For this review, take the finished solid that the model builds, in its own axes (mm). Coordinates: 2 decimals unless noted, no trailing zeros. Write each loop counter-clockwise with the first axis right and the second up, starting at its lowest first coordinate (ties: lowest second). Pieces come first, ordered by that corner, then holes. Notation, with made-up numbers: M 23,-6.5 L 32,-6.5 A23 ccw 32,21.5 Z; hole C 1.5,53.25 d8. An arc over 180 degrees is marked long. Return JSON: item names as keys, results as strings.
```python
from build123d import *

# Parameters (mm, degrees)
F1_DEPTH      = 12.7
F2_R          = 2.3789042868
F3_DEPTH      = 31.75
F3_DEPTH_BACK = 138.176
F4_R          = 5.08
F5_T4_ANGLE   = 90
F5_S5_R       = 2.3789042868
F5_T6_DEPTH   = 6
F5_T10_DEPTH  = 20.32
F5_S11_R      = 2.3789042868
F5_T12_DEPTH  = 12
F5_T16_DEPTH  = 16.390593442
F5_S17_R      = 2.3789042868
F5_T18_DEPTH  = 10
F6_T1_DEPTH   = 113.968887086
F6_T6_ANGLE   = 90.0000000017
F6_S7_R       = 2.3789042868
F6_T8_DEPTH   = 6
F6_T12_DEPTH  = 16.390593442
F6_S13_R      = 2.3789042868
F6_T14_DEPTH  = 10
F7_R          = 1.2458673334
F8_DEPTH      = 25.4
F9_T4_DEPTH   = 16.390593442
F9_S5_R       = 2.3789042868
F9_T6_DEPTH   = 10
F9_T10_DEPTH  = 16.390593442
F9_S11_R      = 2.3789042868
F9_T12_DEPTH  = 10
F9_T16_ANGLE  = 90
F9_S17_R      = 2.3789042868
F9_T18_DEPTH  = 6
F9_T22_DEPTH  = 2.54
F9_S23_R      = 2.3789042868
F9_T24_DEPTH  = 5
F9_T28_ANGLE  = 90.0000000017
F9_S29_R      = 2.3789042868
F9_T30_DEPTH  = 6
F10_R         = 1.24587
F11_DEPTH     = 25.4


# Not quite as in the source:
# - a fillet or chamfer that OpenCascade refuses, or shapes differently, is made with other operations: its cross-section is extruded or revolved along the edge and cut away or added


with BuildPart() as f1:
    # F0 (on Front) → F1 (new body)
    with BuildSketch(Plane.XZ):
        with BuildLine():
            Line((-53.174443543, 7.5021637604), (0, 7.5021637604))
            Line((0, 7.5021637604), (53.174443543, 7.5021637604))
            Line((53.174443543, 7.5021637604), (53.174443543, 16.2727572024))
            Line((53.174443543, 16.2727572024), (27.8020980501, 20.4710588867))
            add(Edge.make_bspline(
                [(27.8020980501, 20.4710588867), (23.5634737704, 22.8817989501), (13.8731335003, 28.3932314282), (12.3127368707, 44.1452356637), (11.4348689094, 53.0072003603)],
                knots=[0, 0, 0, 0, 0.4374071665, 1, 1, 1, 1], degree=3))
            Line((11.4348689094, 53.0072003603), (1.8664607778, 53.0072003603))
            Line((1.8664607778, 53.0072003603), (0, 52.8586618602))
            Line((0, 52.8586618602), (-1.8664607778, 53.0072003603))
            Line((-1.8664607778, 53.0072003603), (-11.4348689094, 53.0072003603))
            add(Edge.make_bspline(
                [(-27.8020980501, 20.4710588867), (-23.5634737704, 22.8817989501), (-13.8731335003, 28.3932314282), (-12.3127368707, 44.1452356637), (-11.4348689094, 53.0072003603)],
                knots=[0, 0, 0, 0, 0.4374071665, 1, 1, 1, 1], degree=3))
            Line((-27.8020980501, 20.4710588867), (-53.174443543, 16.2727572024))
            Line((-53.174443543, 16.2727572024), (-53.174443543, 7.5021637604))
        make_face()
    extrude(amount=F1_DEPTH)

    # F2 (on face) → F3 (join, two sides)
    with BuildSketch(Plane(origin=(-53.174443543, 0, 0), x_dir=(0, -1, 0), z_dir=(-1, 0, 0))) as f3_sk:
        with Locations((6.3686654903, 12.1966870502)):
            Circle(F2_R)
    extrude(amount=F3_DEPTH)
    extrude(f3_sk.sketch, amount=-F3_DEPTH_BACK)

    # F4
    f4_edges = [f1.edges().sort_by_distance(p)[0] for p in [
        (0, 0, 7.502164),
    ]]
    fillet(f4_edges, radius=F4_R)

    # F5: fillet of radius 5.08 on 1 edges, made by hand


with BuildPart() as f5_tool2:
    # F5_s3 → F5_t4 (revolve)
    with BuildSketch(Plane.XZ.offset(5.08)):
        with BuildLine():
            ThreePointArc((-53.174443543, 12.5821637604), (-51.6865459914, 8.9900613119), (-48.094443543, 7.5021637604))
            Line((-48.094443543, 7.5021637604), (-53.174443543, 7.5021637604))
            Line((-53.174443543, 7.5021637604), (-53.174443543, 12.5821637604))
        make_face()
    revolve(axis=Axis((-53.174443543, -5.08, 12.5821637604), (1, 0, 0)), revolution_arc=F5_T4_ANGLE)

    # F5_s5 → F5_t6 (cut, symmetric)
    with BuildSketch(Plane.YZ.offset(-50.6)):
        with Locations((-6.3686654903, 12.1966870502)):
            Circle(F5_S5_R)
    extrude(amount=F5_T6_DEPTH, both=True, mode=Mode.SUBTRACT)


with BuildPart() as f1_1:
    add(f1.part)

    # F5_t1: cut F5_tool2
    add(f5_tool2.part, mode=Mode.SUBTRACT)


with BuildPart() as f5_tool8:
    # F5_s9 → F5_t10 (new body)
    with BuildSketch(Plane.XZ.offset(5.08)):
        with BuildLine():
            ThreePointArc((-48.094443543, 7.5021637604), (-51.6865459914, 8.9900613119), (-53.174443543, 12.5821637604))
            Line((-53.174443543, 12.5821637604), (-53.174443543, 7.5021637604))
            Line((-53.174443543, 7.5021637604), (-48.094443543, 7.5021637604))
        make_face()
    extrude(amount=F5_T10_DEPTH)

    # F5_s11 → F5_t12 (cut, symmetric)
    with BuildSketch(Plane.YZ.offset(-50.6)):
        with Locations((-6.3686654903, 12.1966870502)):
            Circle(F5_S11_R)
    extrude(amount=F5_T12_DEPTH, both=True, mode=Mode.SUBTRACT)


with BuildPart() as f1_2:
    add(f1_1.part)

    # F5_t7: cut F5_tool8
    add(f5_tool8.part, mode=Mode.SUBTRACT)


with BuildPart() as f5_tool14:
    # F5_s15 → F5_t16 (new body)
    with BuildSketch(Plane.XY.offset(28.9727572024)):
        with BuildLine():
            ThreePointArc((-53.174443543, -5.08), (-51.6865459914, -1.4878975516), (-48.094443543, 0))
            Line((-48.094443543, 0), (-53.174443543, 0))
            Line((-53.174443543, 0), (-53.174443543, -5.08))
        make_face()
    extrude(amount=-F5_T16_DEPTH)

    # F5_s17 → F5_t18 (cut, symmetric)
    with BuildSketch(Plane.YZ.offset(-50.6)):
        with Locations((-6.3686654903, 12.1966870502)):
            Circle(F5_S17_R)
    extrude(amount=F5_T18_DEPTH, both=True, mode=Mode.SUBTRACT)


with BuildPart() as f1_3:
    add(f1_2.part)

    # F5_t13: cut F5_tool14
    add(f5_tool14.part, mode=Mode.SUBTRACT)

    # F6: fillet of radius 5.08 on 1 edges, made by hand

    # F6_s2 → F6_t1 (cut)
    with BuildSketch(Plane.YZ.offset(-48.094443543)):
        with BuildLine():
            ThreePointArc((-7.62, 7.5021637604), (-11.2121024484, 8.9900613119), (-12.7, 12.5821637604))
            Line((-12.7, 12.5821637604), (-12.7, 7.5021637604))
            Line((-12.7, 7.5021637604), (-7.62, 7.5021637604))
        make_face()
    extrude(amount=F6_T1_DEPTH, mode=Mode.SUBTRACT)


with BuildPart() as f6_tool4:
    # F6_s5 → F6_t6 (revolve)
    with BuildSketch(Plane.YZ.offset(-48.0944435431)):
        with BuildLine():
            ThreePointArc((-12.7, 12.5821637604), (-11.2121024484, 8.990061312), (-7.62, 7.5021637604))
            Line((-7.62, 7.5021637604), (-12.7, 7.5021637604))
            Line((-12.7, 7.5021637604), (-12.7, 12.5821637604))
        make_face()
    revolve(axis=Axis((-48.0944435431, -12.7, 12.5821637603), (0, 1, 0)), revolution_arc=F6_T6_ANGLE)

    # F6_s7 → F6_t8 (cut, symmetric)
    with BuildSketch(Plane.YZ.offset(-50.6)):
        with Locations((-6.3686654903, 12.1966870502)):
            Circle(F6_S7_R)
    extrude(amount=F6_T8_DEPTH, both=True, mode=Mode.SUBTRACT)


with BuildPart() as f1_4:
    add(f1_3.part)

    # F6_t3: cut F6_tool4
    add(f6_tool4.part, mode=Mode.SUBTRACT)


with BuildPart() as f6_tool10:
    # F6_s11 → F6_t12 (new body)
    with BuildSketch(Plane.XY.offset(28.9727572024)):
        with BuildLine():
            ThreePointArc((-48.094443543, -12.7), (-51.6865459914, -11.2121024484), (-53.174443543, -7.62))
            Line((-53.174443543, -7.62), (-53.174443543, -12.7))
            Line((-53.174443543, -12.7), (-48.094443543, -12.7))
        make_face()
    extrude(amount=-F6_T12_DEPTH)

    # F6_s13 → F6_t14 (cut, symmetric)
    with BuildSketch(Plane.YZ.offset(-50.6)):
        with Locations((-6.3686654903, 12.1966870502)):
            Circle(F6_S13_R)
    extrude(amount=F6_T14_DEPTH, both=True, mode=Mode.SUBTRACT)


with BuildPart() as f1_5:
    add(f1_4.part)

    # F6_t9: cut F6_tool10
    add(f6_tool10.part, mode=Mode.SUBTRACT)

    # F7 (on face) → F8 (cut)
    with BuildSketch(Plane(origin=(-84.924443543, 0, 0), x_dir=(0, -1, 0), z_dir=(-1, 0, 0))):
        with Locations((6.3686654903, 12.1966870502)):
            Circle(F7_R)
    extrude(amount=-F8_DEPTH, mode=Mode.SUBTRACT)

    # F9: fillet of radius 5.08 on 2 edges, made by hand


with BuildPart() as f9_tool2:
    # F9_s3 → F9_t4 (new body)
    with BuildSketch(Plane.XY.offset(12.5821637604)):
        with BuildLine():
            ThreePointArc((53.174443543, -7.62), (51.6865459914, -11.2121024484), (48.094443543, -12.7))
            Line((48.094443543, -12.7), (53.174443543, -12.7))
            Line((53.174443543, -12.7), (53.174443543, -7.62))
        make_face()
    extrude(amount=F9_T4_DEPTH)

    # F9_s5 → F9_t6 (cut, symmetric)
    with BuildSketch(Plane.YZ.offset(50.6)):
        with Locations((-6.3686654903, 12.1966870502)):
            Circle(F9_S5_R)
    extrude(amount=F9_T6_DEPTH, both=True, mode=Mode.SUBTRACT)


with BuildPart() as f1_6:
    add(f1_5.part)

    # F9_t1: cut F9_tool2
    add(f9_tool2.part, mode=Mode.SUBTRACT)


with BuildPart() as f9_tool8:
    # F9_s9 → F9_t10 (new body)
    with BuildSketch(Plane.XY.offset(12.5821637604)):
        with BuildLine():
            ThreePointArc((53.174443543, -5.08), (51.6865459914, -1.4878975516), (48.094443543, 0))
            Line((48.094443543, 0), (53.174443543, 0))
            Line((53.174443543, 0), (53.174443543, -5.08))
        make_face()
    extrude(amount=F9_T10_DEPTH)

    # F9_s11 → F9_t12 (cut, symmetric)
    with BuildSketch(Plane.YZ.offset(50.6)):
        with Locations((-6.3686654903, 12.1966870502)):
            Circle(F9_S11_R)
    extrude(amount=F9_T12_DEPTH, both=True, mode=Mode.SUBTRACT)


with BuildPart() as f1_7:
    add(f1_6.part)

    # F9_t7: cut F9_tool8
    add(f9_tool8.part, mode=Mode.SUBTRACT)


with BuildPart() as f9_tool14:
    # F9_s15 → F9_t16 (revolve)
    with BuildSketch(Plane.XZ.offset(5.08)):
        with BuildLine():
            ThreePointArc((48.094443543, 7.5021637604), (51.6865459914, 8.9900613119), (53.174443543, 12.5821637604))
            Line((53.174443543, 12.5821637604), (53.174443543, 7.5021637604))
            Line((53.174443543, 7.5021637604), (48.094443543, 7.5021637604))
        make_face()
    revolve(axis=Axis((53.174443543, -5.08, 12.5821637604), (1, 0, 0)), revolution_arc=F9_T16_ANGLE)

    # F9_s17 → F9_t18 (cut, symmetric)
    with BuildSketch(Plane.YZ.offset(50.6)):
        with Locations((-6.3686654903, 12.1966870502)):
            Circle(F9_S17_R)
    extrude(amount=F9_T18_DEPTH, both=True, mode=Mode.SUBTRACT)


with BuildPart() as f1_8:
    add(f1_7.part)

    # F9_t13: cut F9_tool14
    add(f9_tool14.part, mode=Mode.SUBTRACT)


with BuildPart() as f9_tool20:
    # F9_s21 → F9_t22 (new body)
    with BuildSketch(Plane.XZ.offset(5.08)):
        with BuildLine():
            ThreePointArc((48.094443543, 7.5021637604), (51.6865459914, 8.9900613119), (53.174443543, 12.5821637604))
            Line((53.174443543, 12.5821637604), (53.174443543, 7.5021637604))
            Line((53.174443543, 7.5021637604), (48.094443543, 7.5021637604))
        make_face()
    extrude(amount=F9_T22_DEPTH)

    # F9_s23 → F9_t24 (cut, symmetric)
    with BuildSketch(Plane.YZ.offset(50.6)):
        with Locations((-6.3686654903, 12.1966870502)):
            Circle(F9_S23_R)
    extrude(amount=F9_T24_DEPTH, both=True, mode=Mode.SUBTRACT)


with BuildPart() as f1_9:
    add(f1_8.part)

    # F9_t19: cut F9_tool20
    add(f9_tool20.part, mode=Mode.SUBTRACT)


with BuildPart() as f9_tool26:
    # F9_s27 → F9_t28 (revolve)
    with BuildSketch(Plane.XZ.offset(7.6200000001)):
        with BuildLine():
            ThreePointArc((53.174443543, 12.5821637604), (51.6865459914, 8.990061312), (48.094443543, 7.5021637604))
            Line((48.094443543, 7.5021637604), (53.174443543, 7.5021637604))
            Line((53.174443543, 7.5021637604), (53.174443543, 12.5821637604))
        make_face()
    revolve(axis=Axis((53.174443543, -7.6200000001, 12.5821637603), (-1, 0, 0)), revolution_arc=F9_T28_ANGLE)

    # F9_s29 → F9_t30 (cut, symmetric)
    with BuildSketch(Plane.YZ.offset(50.6)):
        with Locations((-6.3686654903, 12.1966870502)):
            Circle(F9_S29_R)
    extrude(amount=F9_T30_DEPTH, both=True, mode=Mode.SUBTRACT)


with BuildPart() as f1_10:
    add(f1_9.part)

    # F9_t25: cut F9_tool26
    add(f9_tool26.part, mode=Mode.SUBTRACT)

    # F10 (on face) → F11 (cut)
    with BuildSketch(Plane.YZ.offset(85.001556457)):
        with Locations((-6.3686654903, 12.1966870502)):
            Circle(F10_R)
    extrude(amount=-F11_DEPTH, mode=Mode.SUBTRACT)


solid = f1_10.part
```
1. We need section A-A (x = 4). State the section outline as (y, z) points, plus the area to 3 significant figures.
Checks:
{"outline": "M -12.7,12.58 A5.08 ccw -7.62,7.5 L -5.08,7.5 A5.08 ccw 0,12.58 L 0,53.01 L -12.7,53.01 Z", "area": "567 mm2"}
2. We need section B-B (x = 73.5). State the section outline as (y, z) points, plus the area to 3 significant figures.
Checks:
{"outline": "C -6.37,12.2 d4.76; hole C -6.37,12.2 d2.49", "area": "12.9 mm2"}
3. We need section C-C (x = 39.5). State the section outline as (y, z) points.
Checks:
{"outline": "M -12.7,12.58 A5.08 ccw -7.62,7.5 L -5.08,7.5 A5.08 ccw 0,12.58 L 0,18.54 L -12.7,18.54 Z"}
4. Wall thickness on L1, parallel to Z at x = 72, y = -6.5; L2, parallel to Z at x = 73, y = -7.5; L3, parallel to Y at x = -36.5, z = 12: over which ranges is each line inside the solid? List them lowest first. Write a range as from..to.
Checks:
{"L1": "9.82..10.96, 13.44..14.57", "L2": "10.1..11.67, 12.72..14.29", "L3": "-12.67..-0.03"}
5. Clearance check with flat-ended pins moving along their axes: pin 1 Ø2 at (y, z) = (-6.37, 12.2) entering from +X; pin 2 Ø0.7 at (y, z) = (-6, 12.5) entering from -X; pin 3 Ø5 at (x, y) = (28, -5.5) entering from +Z. State where each tip first meets the part, or that it passes through.
Checks:
{"pin 1": "x = 59.6", "pin 2": "x = -59.52", "pin 3": "z = 21.8"}
